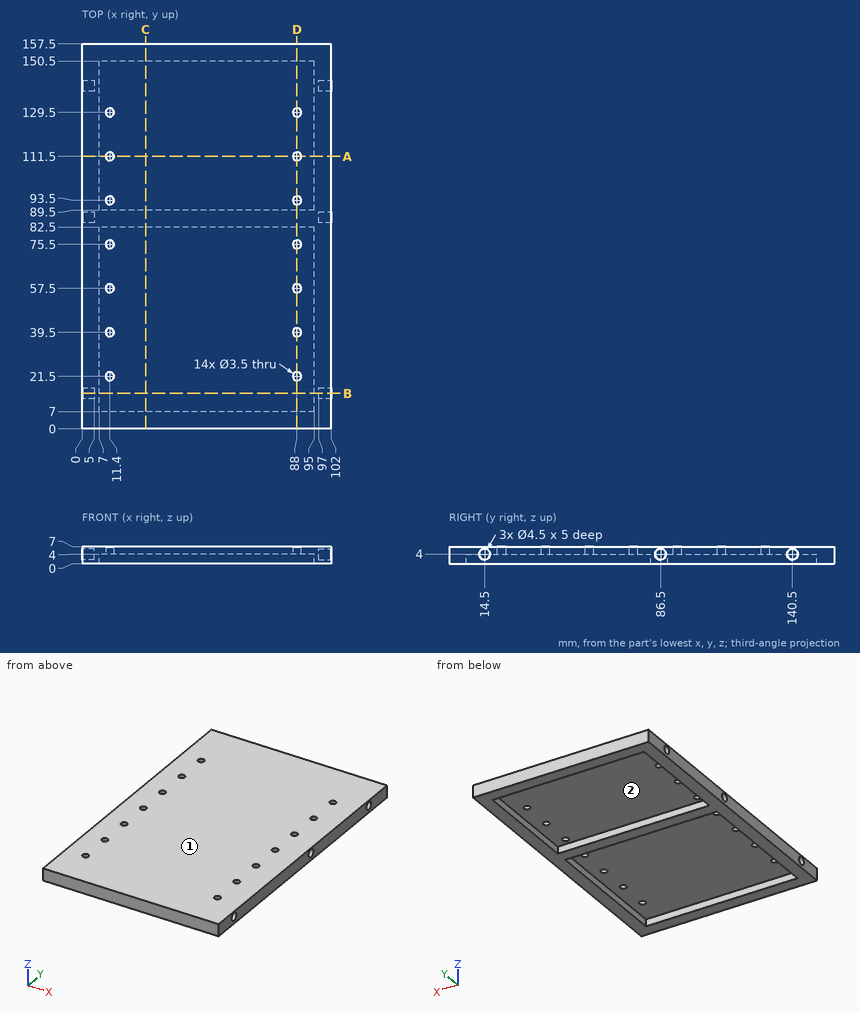
The figure shows three views and two pictorial views of one solid part (mm, origin at its lowest corner). Answer the questions. A direction names the side the tool comes from. Round coordinates to 2 decimals unless told otherwise and drop trailing zeros. Order: outer loops, then holes, each group sorted by start corner. A loop starts at its lowest first (then second) coordinate and runs counter-clockwise, first axis right, second up. Notation, with made-up numbers: (-35.5, -11.5) -> (-27.5, -11.5) arc R22 cw to (-27.5, -3.5) -> close; hole circle Ø7 at (42.25, -37). An arc over 180 degrees is marked (long way). One line per item, written item: value.
Item 1: Given P1, Ø5.5, axis at x = 88, y = 129.5, coming from the -Z side; P2, Ø3.5, axis at y = 86.5, z = 4, coming from the -X side; P3, Ø1.3, axis at y = 141, z = 3.5, coming from the +X side, each flat-ended and moving along its own axis, determine where each tip first touches the part or whether it passes through.
Taken from the geometry:
P1: stops at z = 4
P2: stops at x = 5
P3: stops at x = 97
Item 2: Find section B-B, the plane y = 14.5. Give the vertices of the cut face in (x, z), then the cut area to 3 significant figures.
Taken from the geometry:
outline: (0, 0) -> (7, 0) -> (7, 4) -> (95, 4) -> (95, 0) -> (102, 0) -> (102, 1.75) -> (97, 1.75) -> (97, 6.25) -> (102, 6.25) -> (102, 7) -> (0, 7) -> (0, 6.25) -> (5, 6.25) -> (5, 1.75) -> (0, 1.75) -> close
area: 317 mm2
Item 3: Find section D-D, the plane x = 88. State how many separate pieces and enclosed holes the cut face has, then the cut area to 3 significant figures.
Taken from the geometry:
separate pieces: 8
enclosed holes: 0
area: 483 mm2
Item 4: Straight lines are drawn through the part: L1, parallel to Y at x = 81, z = 2.5; L2, parallel to X at y = 93.5, z = 6.35; L3, parallel to Y at x = 1.5, z = 4. For each, find the intervals that lie inside material, in ascending order.
Taken from the geometry:
L1: y = 0 to 7, 82.5 to 89.5, 150.5 to 157.5
L2: x = 0 to 9.65, 13.15 to 86.25, 89.75 to 102
L3: y = 0 to 12.25, 16.75 to 84.25, 88.75 to 138.25, 142.75 to 157.5
Item 5: Find section C-C, the plane x = 26. Give the vertices of the cut face in (y, z), then the cut area to 4 significant figures.
Taken from the geometry:
outline: (0, 0) -> (7, 0) -> (7, 4) -> (82.5, 4) -> (82.5, 0) -> (89.5, 0) -> (89.5, 4) -> (150.5, 4) -> (150.5, 0) -> (157.5, 0) -> (157.5, 7) -> (0, 7) -> close
area: 556.5 mm2
Item 6: Find section A-A, the plane y = 111.5. Give the vertices of the cut face in (x, z).
Taken from the geometry:
outline: (0, 0) -> (7, 0) -> (7, 4) -> (9.65, 4) -> (9.65, 7) -> (0, 7) -> close; (13.15, 4) -> (86.25, 4) -> (86.25, 7) -> (13.15, 7) -> close; (89.75, 4) -> (95, 4) -> (95, 0) -> (102, 0) -> (102, 7) -> (89.75, 7) -> close
Item 7: For the marked faces 1 and 2, determine the directions among +Z, -Z, +X, -X, +Y, -Y from which every point of the face is accessible in a straight line to the end or side of a thin tool.
Taken from the geometry:
face 1: +Z, +X, -X, +Y, -Y
face 2: -Z
